```python
from build123d import *

# Parameters (mm, degrees)
BOSS_EXTRUDE1_DEPTH  = 5
SKETCH3_W            = 4
SKETCH3_H            = 5
BOSS_EXTRUDE2_DEPTH  = 3
SKETCH4_R            = 1.08
CUT_EXTRUDE1_DEPTH   = 6
LPATTERN1_COUNT      = 2
LPATTERN1_PITCH      = 60
LPATTERN1_COUNT_DIR2 = 2
LPATTERN1_PITCH_DIR2 = 82
LPATTERN2_COUNT      = 2
LPATTERN2_PITCH      = 60
LPATTERN2_COUNT_DIR2 = 2
LPATTERN2_PITCH_DIR2 = 82
SKETCH5_W            = 3
SKETCH5_H            = 4
CUT_EXTRUDE2_DEPTH   = 4
CUT_EXTRUDE3_DEPTH   = 4
FILLET1_R            = 2


with BuildPart() as part:
    # Sketch2 → Boss-Extrude1 (new body)
    with BuildSketch(Plane(origin=(0, 0, 0), x_dir=(1, 0, 0), z_dir=(0, 1, 0))):
        Polygon((0, 0), (79, 0), (79, 70), (0, 70), (0, 50), (15, 50), (15, 30), (0, 30), align=None)
    extrude(amount=BOSS_EXTRUDE1_DEPTH)

    # Sketch3 → Boss-Extrude2 (add)
    with BuildSketch(Plane(origin=(79, 0, 0), x_dir=(0, 0, -1), z_dir=(1, 0, 0))):
        with Locations((5, 2.5)):
            Rectangle(SKETCH3_W, SKETCH3_H)
    boss_extrude2 = extrude(amount=BOSS_EXTRUDE2_DEPTH)

    # Sketch4 → Cut-Extrude1 (cut, through all)
    with BuildSketch(Plane(origin=(0, 5, 0), x_dir=(1, 0, 0), z_dir=(0, 1, 0))):
        with Locations((80.5, 5)):
            Circle(SKETCH4_R)
    cut_extrude1 = extrude(amount=-CUT_EXTRUDE1_DEPTH, mode=Mode.SUBTRACT)

    # LPattern1: Boss-Extrude2 2 × 2
    with Locations(*[(-j * LPATTERN1_PITCH_DIR2, 0, -i * LPATTERN1_PITCH) for i in range(LPATTERN1_COUNT) for j in range(LPATTERN1_COUNT_DIR2) if (i, j) != (0, 0)]):
        add(boss_extrude2)

    # LPattern2: Cut-Extrude1 2 × 2
    with Locations(*[(-j * LPATTERN2_PITCH_DIR2, 0, -i * LPATTERN2_PITCH) for i in range(LPATTERN2_COUNT) for j in range(LPATTERN2_COUNT_DIR2) if (i, j) != (0, 0)]):
        add(cut_extrude1, mode=Mode.SUBTRACT)

    # Sketch5 → Cut-Extrude2 (cut)
    with BuildSketch(Plane(origin=(0, 5, 0), x_dir=(1, 0, 0), z_dir=(0, 1, 0))):
        with Locations((-1.5, 65)):
            Rectangle(SKETCH5_W, SKETCH5_H)
        with Locations((-1.5, 5)):
            Rectangle(SKETCH5_W, SKETCH5_H)
        with Locations((80.5, 5)):
            Rectangle(SKETCH5_W, SKETCH5_H)
        with Locations((80.5, 65)):
            Rectangle(SKETCH5_W, SKETCH5_H)
    extrude(amount=-CUT_EXTRUDE2_DEPTH, mode=Mode.SUBTRACT)

    # Sketch7 → Cut-Extrude3 (cut)
    with BuildSketch(Plane.XZ):
        Polygon((2, -2), (77, -2), (77, -68), (2, -68), (2, -52), (17, -52), (17, -28), (2, -28), align=None)
    extrude(amount=-CUT_EXTRUDE3_DEPTH, mode=Mode.SUBTRACT)

    # Fillet1
    fillet1_edges = [part.edges().sort_by_distance(p)[0] for p in [
        (79, 5, -35),
        (39.5, 5, -70),
        (0, 5, -60),
        (7.5, 5, -50),
        (15, 5, -40),
        (7.5, 5, -30),
        (0, 5, -15),
        (39.5, 5, 0),
    ]]
    fillet(fillet1_edges, radius=FILLET1_R)


solid = part.part
```
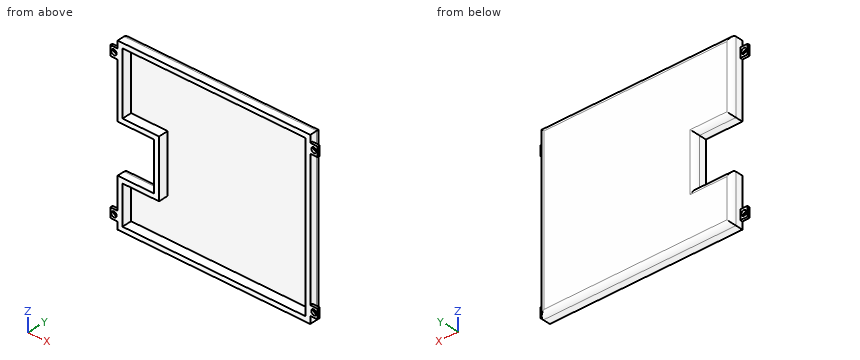
Geometry: final body of the model. Coordinates: model frame, mm. Round coordinates to 2 decimals unless told otherwise and drop trailing zeros. Order: outer loops, then holes, each group sorted by start corner. A loop starts at its lowest first (then second) coordinate and runs counter-clockwise, first axis right, second up. Notation, with made-up numbers: M -39.75,20 L 13.25,20 A28 cw 13.25,57 Z; hole C 65,-23 d7. An arc over 180 degrees is marked long. One line per item, written item: value.
(1) Line query: probe 1 along X at (y, z) = (0.7, -5); probe 2 along Z at (x, y) = (-1.5, 0.6); probe 3 along X at (y, z) = (1.55, -66). Output: solid intervals per line, ascending. Write a range as [from, to].
Result sheet:
probe 1: [-3, -2.58], [-0.42, 2], [77, 79.42], [81.58, 82]
probe 2: [-67, -66.08], [-63.92, -63], [-7, -6.08], [-3.92, -3]
probe 3: [0, 2], [77, 79]
(2) Cut plane B-B (z = -5). Return the cut outline in (x, y), and give its area (3 significant figures).
Result sheet:
outline: M -3,0 L -2.58,0 L -2.58,1 L -3,1 Z; M -0.42,0 L 2,0 L 2,4 L 77,4 L 77,0 L 79.42,0 L 79.42,1 L 79,1 L 79,3 A2 ccw 77,5 L 2,5 A2 ccw 0,3 L 0,1 L -0.42,1 Z; M 81.58,0 L 82,0 L 82,1 L 81.58,1 Z
area: 95.0 mm2
(3) Cut plane D-D (x = 69). Return the cut outline in (y, z).
Result sheet:
outline: M 0,-70 L 3,-70 A2 ccw 5,-68 L 5,-2 A2 ccw 3,0 L 0,0 L 0,-2 L 4,-2 L 4,-68 L 0,-68 Z
(4) Cut plane A-A (x = 80.5). Return the cut outline in (y, z), and give its area (3 significant figures).
Result sheet:
outline: M 0,-67 L 1,-67 L 1,-66.08 L 0,-66.08 Z; M 0,-63.92 L 1,-63.92 L 1,-63 L 0,-63 Z; M 0,-7 L 1,-7 L 1,-6.08 L 0,-6.08 Z; M 0,-3.92 L 1,-3.92 L 1,-3 L 0,-3 Z
area: 3.68 mm2
(5) Pin query (flat end, axial travel): P1, Ø1.5, axis at x = 32, y = 4, coming from the +Z side; P2, Ø1.9, axis at x = -1.5, z = -5, coming from the +Y side; P3, Ø1.2, axis at y = 1, z = -18, coming from the +X side; P4, Ø1.5, axis at x = 81, z = -64.5, coming from the +Y side. Return the tip coordinate at first contact, or that it passes through.
Result sheet:
P1: z = -0.02
P2: through
P3: x = 79
P4: y = 1
(6) Cut plane C-C (z = -59). Return the cut outline in (x, y).
Result sheet:
outline: M 0,0 L 2,0 L 2,4 L 77,4 L 77,0 L 79,0 L 79,3 A2 ccw 77,5 L 2,5 A2 ccw 0,3 Z
